from build123d import *

# Parameters (mm, degrees)
SKETCH1_W                    = 100
SKETCH1_H                    = 46
BOSS_EXTRUDE1_DEPTH          = 6
TAP_DRILL_FOR_M3_TAP1_D      = 2.5
TAP_DRILL_FOR_M5_HELICOIL1_D = 5.2


with BuildPart() as part:
    # Sketch1 → Boss-Extrude1 (new body)
    with BuildSketch(Plane(origin=(0, 0, 0), x_dir=(1, 0, 0), z_dir=(0, 1, 0))):
        with Locations((50, 23)):
            Rectangle(SKETCH1_W, SKETCH1_H)
    extrude(amount=BOSS_EXTRUDE1_DEPTH)

    # Tap Drill for M3 Tap1 (through all)
    with Locations(Plane(origin=(0, 0, -46), x_dir=(-1, 0, 0), z_dir=(0, 0, -1))):
        with Locations((-90, 3), (-70, 3), (-50, 3), (-30, 3), (-10, 3)):
            Hole(TAP_DRILL_FOR_M3_TAP1_D / 2)

    # Tap Drill for M5 Helicoil1 (through all)
    with Locations(Plane(origin=(0, 6, 0), x_dir=(1, 0, 0), z_dir=(0, 1, 0))):
        with Locations((30.5, 24), (69.5, 24)):
            Hole(TAP_DRILL_FOR_M5_HELICOIL1_D / 2)


solid = part.part
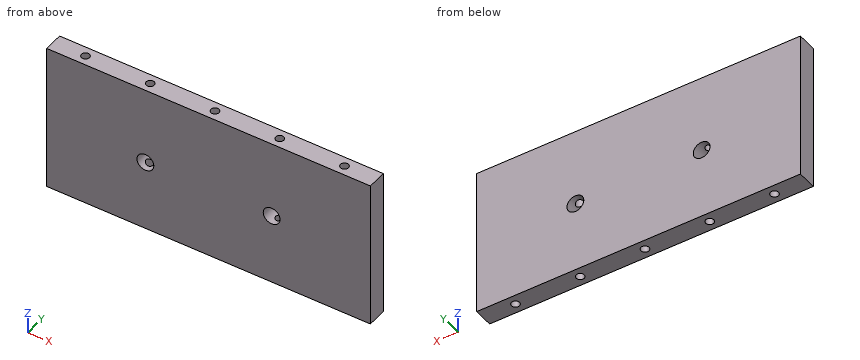
For this review, take the finished solid that the model builds, in its own axes (mm). Coordinates: 2 decimals unless noted, no trailing zeros. Order: outer loops, then holes, each group sorted by start corner. A loop starts at its lowest first (then second) coordinate and runs counter-clockwise, first axis right, second up. Notation, with made-up numbers: (-1, 29) - (56, 29) arc R27 cw to (56, 64) - close; hole circle Ø6 at (51.25, -23). An arc over 180 degrees is marked (long way). Answer as CSV lines item,"result". Start each with the question number.
1) Add section C-C (y = 3). Count the separate pieces of the cut face and the enclosed holes in it, then the cut area to 3 significant figures.
2) Add section D-D (x = 70). State the section outline as (y, z) points.
3) Add section B-B (z = -35). State the section outline as (x, y) points, then the cut area to 3 significant figures.
4) To check wall thickness, follow line 1 along Y through (x, z) = (90, -34); line 2 along Z through (x, y) = (30.5, 4.75); line 3 along X through (y, z) = (2, -16.5). State the ranges of each line that lie inside material, in increasing order. Write a range as [from, to].
5) Add section A-A (z = -24). State the section outline as (x, y) points.
Result:
1,separate pieces,"6"
1,enclosed holes,"0"
1,area,"4,010 mm^2"
2,outline,"(0, -46) - (1.75, -46) - (1.75, -26.55) - (0, -26.55) - close; (0, -21.45) - (1.75, -21.45) - (1.75, 0) - (0, 0) - close; (4.25, -46) - (6, -46) - (6, -26.55) - (4.25, -26.55) - close; (4.25, -21.45) - (6, -21.45) - (6, 0) - (4.25, 0) - close"
3,outline,"(0, 0) - (100, 0) - (100, 6) - (0, 6) - close; hole circle Ø2.5 at (10, 3); hole circle Ø2.5 at (30, 3); hole circle Ø2.5 at (50, 3); hole circle Ø2.5 at (70, 3); hole circle Ø2.5 at (90, 3)"
3,area,"575 mm^2"
4,line 1,"[0, 1.75], [4.25, 6]"
4,line 2,"[-46, -26.6], [-21.4, 0]"
4,line 3,"[0, 9.25], [10.75, 29.25], [30.75, 49.25], [50.75, 69.25], [70.75, 89.25], [90.75, 100]"
5,outline,"(0, 0) - (27.9, 0) - (27.9, 6) - (0, 6) - close; (33.1, 0) - (66.9, 0) - (66.9, 6) - (33.1, 6) - close; (72.1, 0) - (100, 0) - (100, 6) - (72.1, 6) - close; hole circle Ø2.5 at (10, 3); hole circle Ø2.5 at (50, 3); hole circle Ø2.5 at (90, 3)"
